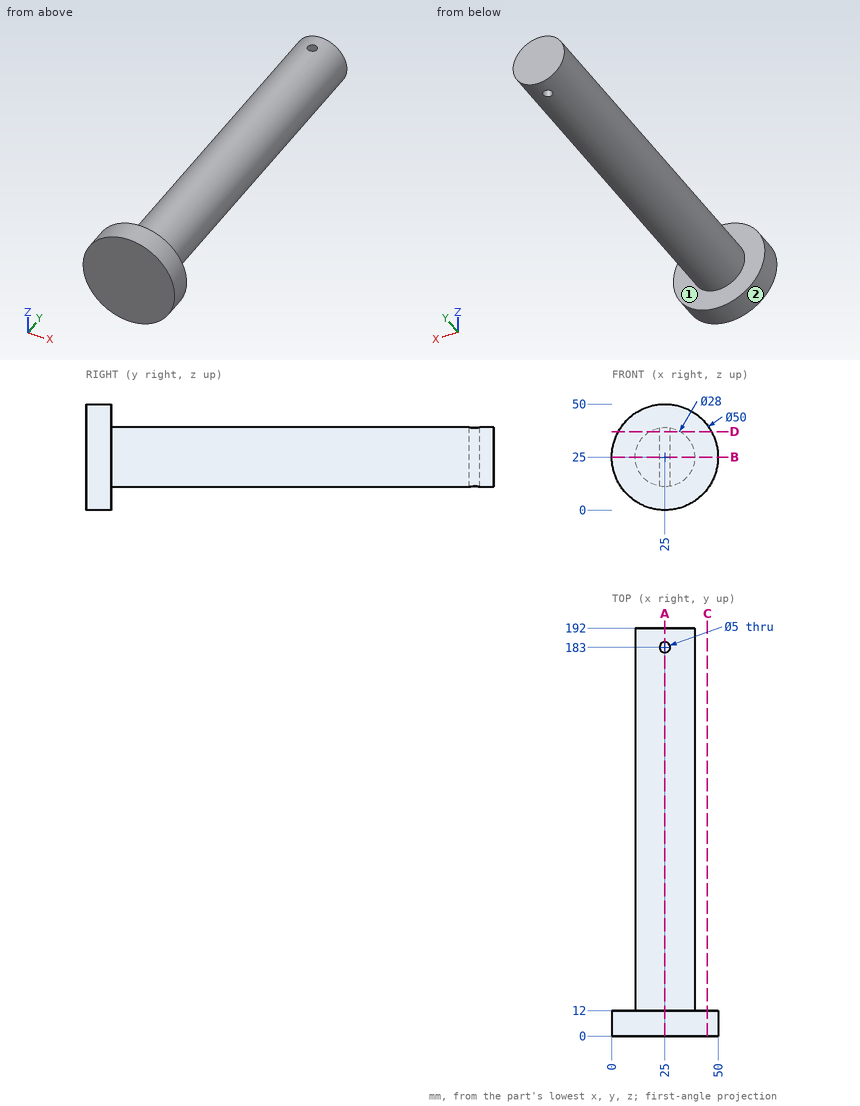
Job drawing, mm, ordinate dimensions from the low corner. One solid piece. A direction names the side the tool comes from. Give positions to 0.01 mm unless a question says otherwise; leave off trailing zeros. Loops run counter-clockwise (first coordinate to the right, second up) from the corner with the lowest first, then second, coordinate; pieces in that order, holes last. Notation, with made-up numbers: (-22.5, -32) -> (11.5, -32) arc R11 cw to (11.5, -25) -> close; hole circle Ø9 at (-26, 57). An arc over 180 degrees is marked (long way). Use a Markdown table: item, result. Add a question column.
(1) Slice it at B-B on z = 25. List the corners of the cut face in (x, y).
(2) Wall check: line 1 along Y through (x, z) = (25, 17); line 2 along X through (y, z) = (183, 25); line 3 along Y through (x, z) = (34, 37.5). Give the ranges that are in metal, low to high.
(3) Tool access for the marked faces 1 and 2: list every direction of +Z, -Z, +X, -X, +Y, -Y with a clear straight run to the whole face (end or side of a thin tool).
(4) Slice it at D-D on z = 37. List the corners of the cut face in (x, y).
(5) Slice it at C-C on x = 45. List the corners of the cut face in (y, z), and give its area (3 significant figures).
(6) Drop flat-ended pins along their axis: pin 1 Ø3 at (x, z) = (12, 5.5) entering from +Y; pin 2 Ø6.5 at (x, y) = (25, 183) entering from -Z; pin 3 Ø12 at (x, y) = (33.5, 56.5) entering from +Z (3 decimals). Give the stop position or say it passes through.
(7) Slice it at A-A on x = 25. List the corners of the cut face in (y, z), and give its area (3 significant figures).
Filled sheet:
| question | item | result |
|---|---|---|
| 1 | outline | (0, 0) -> (50, 0) -> (50, 12) -> (39, 12) -> (39, 192) -> (11, 192) -> (11, 12) -> (0, 12) -> close; hole circle Ø5 at (25, 183) |
| 2 | line 1 | 0 to 180.5, 185.5 to 192 |
| 2 | line 2 | 11 to 22.5, 27.5 to 39 |
| 2 | line 3 | 0 to 12 |
| 3 | face 1 | +Y |
| 3 | face 2 | +Y, -Y |
| 4 | outline | (3.07, 0) -> (46.93, 0) -> (46.93, 12) -> (32.21, 12) -> (32.21, 192) -> (17.79, 192) -> (17.79, 12) -> (3.07, 12) -> close; hole circle Ø5 at (25, 183) |
| 5 | outline | (0, 10) -> (12, 10) -> (12, 40) -> (0, 40) -> close |
| 5 | area | 360 mm2 |
| 6 | pin 1 | y = 12 |
| 6 | pin 2 | z = 11 |
| 6 | pin 3 | z = 38.775 |
| 7 | outline | (0, 0) -> (12, 0) -> (12, 11) -> (180.5, 11) -> (180.5, 39) -> (12, 39) -> (12, 50) -> (0, 50) -> close; (185.5, 11) -> (192, 11) -> (192, 39) -> (185.5, 39) -> close |
| 7 | area | 5,500 mm2 |
